Geometry: final body of the model. Coordinates: model frame, mm. A direction names the side the tool comes from. Coordinates: 2 decimals unless noted, no trailing zeros. Write each loop counter-clockwise with the first axis right and the second up, starting at its lowest first coordinate (ties: lowest second). Pieces come first, ordered by that corner, then holes.
Autodesk Inventor part; units mm, degrees
ref_plane "YZ Plane" through (0, 0, 0) normal (1, 0, 0) x (0, 1, 0)
ref_plane "XZ Plane" through (0, 0, 0) normal (0, 1, 0) x (-1, 0, 0)
ref_plane "XY Plane" through (0, 0, 0) normal (0, 0, 1) x (1, 0, 0)
ref_plane "Work Plane1" through (0, 0, 2) normal (0, 0, 1) x (1, 0, 0)
sketch "Sketch1" plane through (0, 0, 2) normal (0, 0, 1) x (1, 0, 0)
  line L0 (-37.0712, 14) -> (-9.0712, 14) construction
  line L1 (-9.0712, 14) -> (-9.0712, -14) construction
  line L2 (-9.0712, -14) -> (-37.0712, -14) construction
  line L3 (-37.0712, -14) -> (-37.0712, 14) construction
  line L4 (-4.0712, -19) -> (-4.0712, 19)
  line L5 (-4.0712, 19) -> (-42.0712, 19)
  line L6 (-42.0712, 19) -> (-42.0712, -19)
  line L7 (-42.0712, -19) -> (-4.0712, -19)
  circle A0 centre (-23.0712, 0) radius 12.8
  point P0 (0, 0)
  dimension "d0" = 5
extrude "Extrusion1" add sketch "Sketch1" along normal blind 9.3 contours L7 L6 L5 L4 | A0
sketch "Sketch3" plane through (0, 0, 2) normal (0, 0, -1) x (-1, 0, 0)
  circle A0 centre (9.0712, -14) radius 1.45 construction
  circle A1 centre (9.0712, -14) radius 2.45
  circle A2 centre (37.0712, -14) radius 1.45
  circle A3 centre (37.0712, -14) radius 1.95
  point P0 (0, 0)
  dimension "d8" = 1
  dimension "d10" = 0.5
chamfer "Chamfer1" distance 3 angle 45 4 edges at (-42.0712, 19, 6.65) (-4.0712, 19, 6.65) (-4.0712, -19, 6.65) (-42.0712, -19, 6.65)
hole "Hole1" at (-37.0712, -14, 2) direction (0, 0, 1) diameter 4 depth 0.1 tip angle 100
sketch "Sketch4" plane through (-4.0712, -19, 2) normal (1, 0, 0) x (0, 0, -1)
  line L0 (2, 4.45) -> (6, 4.45)
  line L1 (2, 1.55) -> (6, 1.55)
  line L2 (0, 0) -> (0, 38)
  arc A0 (2, 19) -> (2, 19) centre (1.5, 4.4206) ccw
  line L3 (-1.7782, 5) -> (-0.1, 7)
  line L4 (-1.7782, 5) -> (-0.1, 3)
  line L5 (-0.1, 7) -> (0.6045, 7)
  line L6 (0.6045, 7) -> (0.6045, 3)
  line L7 (0.6045, 3) -> (-0.1, 3)
  line L8 (-0.1, 3) -> (-0.1, 7)
extrude "Extrusion4" cut sketch "Sketch4" against normal blind 8 contours L7 L8 L5 L2 | L2 L5 L6 L7 | L4 L3 L8
ref_plane "Arbeitsebene2" through (-23.0712, -12, 2) normal (1, 0, 0) x (0, 0, -1)
ref_plane "Arbeitsebene3" through (-39.0712, 0, 2) normal (0, -1, 0) x (1, 0, 0)
sketch "Skizze9" plane through (0, 0, 2) normal (0, 0, -1) x (-1, 0, 0)
  line L0 (12.0712, -16) -> (4.0712, -16)
  line L1 (7.0712, -19) -> (4.0712, -16)
  line L2 (39.0712, -19) -> (7.0712, -19)
  line L3 (42.0712, -16) -> (39.0712, -19)
  line L4 (42.0712, 16) -> (42.0712, -16)
  line L5 (39.0712, 19) -> (42.0712, 16)
  line L6 (7.0712, 19) -> (39.0712, 19)
  line L7 (4.0712, 16) -> (7.0712, 19)
  line L8 (4.0712, -12) -> (4.0712, 16)
  line L9 (4.0712, -12) -> (12.0712, -12)
  line L10 (12.0712, -12) -> (12.0712, -16)
  circle A0 centre (37.0712, -14) radius 2
  circle A1 centre (28.0712, -14) radius 3
  circle A2 centre (9.0712, 5) radius 3
  point P0 (0, 0)
  dimension "d54" = 6
  dimension "d55" = 6
  dimension "d56" = 14
  dimension "d57" = 5
  dimension "d58" = 5
  dimension "d59" = 14
extrude "Extrusion9" cut sketch "Skizze9" against normal blind 3 draft -2 contours A1 | A2
sketch "Skizze10" plane through (0, 0, 11.3) normal (0, 0, 1) x (1, 0, 0)
  circle A0 centre (-9.0712, 5) radius 4.05
  circle A1 centre (-28.0712, -14) radius 4.55
  circle A2 centre (-9.0712, 5) radius 4
  circle A3 centre (-28.0712, -14) radius 2.8952
  circle A4 centre (-28.0712, -14) radius 4
  point P0 (0, 0)
  dimension "d62" = 8
  dimension "d63" = 8
extrude "Extrusion10" cut sketch "Skizze10" against normal blind 8.8 contours A2 | A3 | A4
sketch "Sketch11" plane through (0, 0, 11.3) normal (0, 0, 1) x (1, 0, 0)
  circle A0 centre (-23.0712, 0) radius 12.8
  line L0 (-39.0712, -19) -> (-7.0712, -19)
  line L1 (-42.0712, 16) -> (-42.0712, -16)
  point P0 (0, 0)
  point P1 (-23.0712, -19)
  point P2 (-42.0712, 0)
  dimension "d66" = 25.6
extrude "Extrusion11" cut sketch "Sketch11" against normal blind 5.5
equation "\"d54\" = d55"
equation "\"d59\" = d56"
properties part number "20_Cube_Insert_Kinematic_Astromedia_30x40x1_45_pro_magnetic"
Item 1: Section B-B, the plane y = 5. Output: boundary loops of the cut face in (x, z).
Derived:
outline: (-42.07, 2) - (-12.07, 2) - (-12.05, 2.5) - (-13.07, 2.5) - (-13.07, 5.8) - (-34.85, 5.8) - (-34.85, 11.3) - (-42.07, 11.3) - close; (-6.09, 2.5) - (-6.07, 2) - (-4.07, 2) - (-4.07, 11.3) - (-5.07, 11.3) - (-5.07, 2.5) - close
Item 2: Section C-C, the plane y = 0. Output: boundary loops of the cut face in (x, z).
Derived:
outline: (-42.07, 2) - (-4.07, 2) - (-4.07, 11.3) - (-10.27, 11.3) - (-10.27, 5.8) - (-35.87, 5.8) - (-35.87, 11.3) - (-42.07, 11.3) - close
Item 3: Section A-A, the plane z = 5. Output: boundary loops of the cut face in (x, y), plus the area to 3 significant figures.
Derived:
outline: (-42.07, -16) - (-39.07, -19) - (-7.07, -19) - (-4.07, -16) - (-4.07, 16) - (-7.07, 19) - (-39.07, 19) - (-42.07, 16) - close; hole circle Ø8 at (-28.07, -14); hole circle Ø8 at (-9.07, 5)
area: 1,330 mm2
Item 4: Pin query (flat end, axial travel): pin 1 (4 mm diameter, centred on x = -26, y = -13, fed in from +Z); pin 2 (1.5 mm diameter, centred on x = -35, y = -1, fed in from +Z); pin 3 (0.5 mm diameter, centred on y = -14.5, z = 2.5, fed in from +X); pin 4 (6.5 mm diameter, centred on x = -9.07, y = 5, fed in from +Z). Return the tip coordinate at first contact, or that it passes through.
Derived:
pin 1: stops at z = 11.3
pin 2: stops at z = 5.8
pin 3: stops at x = -12.07
pin 4: stops at z = 2.5
Item 5: Pull-direction query (Y, two-part tool) for faces 4 (the flat face through (-40.55, 17.52, 6.58)), 5 (the flat face through (-42.071, 0, 7)), 6 (the conical face through (-36.73, -14.05, 3.49)); classes: released by +Y, released by -Y, zero draft, split by the parting line, or undercut.
Derived:
face 4: released by +Y
face 5: zero draft
face 6: undercut
Item 6: Section D-D, the plane z = 3. Output: boundary loops of the cut face in (x, y).
Derived:
outline: (-42.07, -16) - (-39.07, -19) - (-7.07, -19) - (-4.07, -16) - (-4.07, -14.93) - (-12.07, -14.93) - (-12.07, -13.07) - (-4.07, -13.07) - (-4.07, 16) - (-7.07, 19) - (-39.07, 19) - (-42.07, 16) - close; hole circle Ø1.85 at (-37.07, -14); hole circle Ø8 at (-28.07, -14); hole circle Ø8 at (-9.07, 5)
Item 7: Material intervals for probe 1 along X at (y, z) = (-14, 2.1); probe 2 along X at (y, z) = (-14, 8.75); probe 3 along Y at (x, z) = (-31, 9.75), sorted ascending.
Derived:
probe 1: x = -42.07 to -39.07, -35.07 to -31.07, -25.07 to -12.07
probe 2: x = -42.07 to -32.07, -24.07 to -4.07
probe 3: y = -19 to -16.72, -11.28 to -10.05, 10.05 to 19
Item 8: Set-up query: faces 1 (the flat face through (-8.02, -13.01, 2.95)), 2 (the flat face through (-30, -17, 2.5)), 3 (the flat face through (-23, 13, 11.3)). Return all of +Z, -Z, +X, -X, +Y, -Y with unobstructed straight access to the full face (end or side cutting, diameter ignored); none if empty.
Derived:
face 1: -Z, +X
face 2: +Z
face 3: +Z, +X, -X, +Y, -Y
